Verification items for the finished model (mm, model axes). A direction names the side the tool comes from. Coordinates: 2 decimals unless noted, no trailing zeros. Order: outer loops, then holes, each group sorted by start corner. A loop starts at its lowest first (then second) coordinate and runs counter-clockwise, first axis right, second up.
Q1. Cross-section at B-B, the plane x = 17. Record the boundary of the cut face in (y, z) (3 decimals), and give its area (3 significant figures).
Q2. Depth check by flat-ended pin: P1, Ø1.5, axis at x = 8.5, z = 108.5, coming from the -Y side; P2, Ø2, axis at x = 19, y = 15, coming from the -Z side; P3, Ø5, axis at x = 23, y = 13.5, coming from the -Z side; P4, Ø12, axis at x = 42.5, y = 18, coming from the -Z side. Enter the tip coordinate at first touch or a pass-through.
Q3. Thickness scan on line 1 (Y direction, x = 7, z = 22); line 2 (Z direction, x = 47, y = 6.75); line 3 (Z direction, x = 14.5, y = 17.25). Record the ranges inside material, lowest first.
Q4. Cross-section at D-D, the plane z = 91.5. Record the boundary of the cut face in (x, y) (3 decimals), and give its area (3 significant figures).
Q5. Set-up check for faces 1 (the flat face through (29, 22.225, 76)), 2 (the cylindrical face through (18.847, 20.615, 99.663)): record each of +Z, -Z, +X, -X, +Y, -Y from which the full face is reachable in a straight line by a thin tool's end or side.
Q6. Cross-section at A-A, the plane z = 76.2. Record the boundary of the cut face in (x, y) (3 decimals).
Q7. Cross-section at C-C, the plane x = 45. Record the boundary of the cut face in (y, z) (3 decimals).
from build123d import *

# Parameters (mm, degrees)
SKETCH2_W           = 57.15
SKETCH2_H           = 152.4
BOSS_EXTRUDE1_DEPTH = 19.05
CUT_EXTRUDE2_DEPTH  = 57.15
SKETCH5_R           = 25.4
BOSS_EXTRUDE2_DEPTH = 3.175


with BuildPart() as part:
    # Sketch2 → Boss-Extrude1 (new body)
    with BuildSketch(Plane(origin=(0, 0, 0), x_dir=(1, 0, 0), z_dir=(0, 1, 0))):
        with Locations((28.575, -76.2)):
            Rectangle(SKETCH2_W, SKETCH2_H)
    extrude(amount=BOSS_EXTRUDE1_DEPTH)

    # Sketch3 → Cut-Extrude2 (cut)
    with BuildSketch(Plane(origin=(57.15, 0, 0), x_dir=(0, 0, -1), z_dir=(1, 0, 0))):
        Polygon((-152.4, 6.447169547), (-139.797169547, 19.05), (-152.4, 19.05), align=None)
        Polygon((0, 6.447169547), (-12.602830453, 19.05), (0, 19.05), align=None)
    extrude(amount=-CUT_EXTRUDE2_DEPTH, mode=Mode.SUBTRACT)

    # Sketch5 → Boss-Extrude2 (add)
    with BuildSketch(Plane(origin=(0, 19.05, 0), x_dir=(1, 0, 0), z_dir=(0, 1, 0))):
        with Locations(Location((28.575, -76.2, 0), (0, 0, 270))):
            Circle(SKETCH5_R)
    extrude(amount=BOSS_EXTRUDE2_DEPTH)


solid = part.part
Check values:
1. outline: (0, 0) - (6.447, 0) - (19.05, 12.603) - (19.05, 53.591) - (22.225, 53.591) - (22.225, 98.809) - (19.05, 98.809) - (19.05, 139.797) - (6.447, 152.4) - (0, 152.4) - close
1. area: 2,890 mm2
2. P1: stops at y = 0
2. P2: stops at z = 7.55
2. P3: stops at z = 4.55
2. P4: stops at z = 5.55
3. line 1: y = 0 to 19.05
3. line 2: z = 0.3 to 152.1
3. line 3: z = 10.8 to 141.6
4. outline: (0, 0) - (57.15, 0) - (57.15, 19.05) - (48.85, 19.05) - (48.85, 22.225) - (8.3, 22.225) - (8.3, 19.05) - (0, 19.05) - close
4. area: 1,220 mm2
5. face 1: +Z, -Z, +X, -X, +Y
5. face 2: +Y
6. outline: (0, 0) - (57.15, 0) - (57.15, 19.05) - (53.975, 19.05) - (53.975, 22.225) - (3.175, 22.225) - (3.175, 19.05) - (0, 19.05) - close
7. outline: (0, 0) - (6.447, 0) - (19.05, 12.603) - (19.05, 56.825) - (22.225, 56.825) - (22.225, 95.575) - (19.05, 95.575) - (19.05, 139.797) - (6.447, 152.4) - (0, 152.4) - close
